Geometry: final body of the model. Coordinates: model frame, mm. A direction names the side the tool comes from. Coordinates: 2 decimals unless noted, no trailing zeros. Loops run counter-clockwise (first coordinate to the right, second up) from the corner with the lowest first, then second, coordinate; pieces in that order, holes last. Notation, with made-up numbers: (68, 7) -> (84, 7) arc R21 cw to (84, 12) -> close; hole circle Ø10 at (29, -8.5). An arc over 180 degrees is marked (long way). One line per item, written item: value. Start each with the question number.
Item 1: Section query C-C on y = 1.75. Return loops of the section in (x, z), then the cut area to 3 significant figures.
Item 2: Ray query, probe 1 along Z at (x, y) = (0.5, 3.5); probe 2 along Z at (x, y) = (1, 1.5); probe 3 along Y at (x, z) = (-1, -41.5). Return the intervals inside material, ascending. Write a range as from..to.
Item 3: Section query B-B on z = 0.5. Return loops of the section in (x, y) (3 decimals).
Item 4: Section query A-A on x = 0. Return loops of the section in (y, z) (3 decimals), then the cut area to 3 significant figures.
Item 5: Mould query, pull axis X, two halves, no side actions, for faces 4 (the flat face through (0, 2.468, 3)), 5 (the flat face through (0, 0, -45)), 6 (the cylindrical face through (2.6, -4.99, 1.97)). Classes: +X half, -X half, draft (parallel to the pull), parting line (faces both ways), or undercut.
Item 6: Contact query for flat-ended pins moving along their axis: pin 1 Ø6 at (x, z) = (-4, -38) entering from -Y; pin 2 Ø5 at (x, z) = (-0.5, -3.5) entering from +Y; pin 3 Ø5 at (y, z) = (-2.5, -38.5) entering from +X. Output: stop coordinate, or through.
Item 7: Set-up query: faces 1 (the flat face through (0, -2.468, 3)), 2 (the flat face through (0, 3, 4)), 3 (the flat face through (2.4, -2.4, 0)). Return all of +Z, -Z, +X, -X, +Y, -Y with unobstructed straight access to the full face (end or side cutting, diameter ignored); none if empty.
Item 8: Section query D-D on z = -9. Return loops of the section in (x, y), then the cut area to 3 significant figures.
from build123d import *

# Parameters (mm, degrees)
ESBO_O1_R                = 5.625
RESSALTO_EXTRUS_O1_DEPTH = 4
CORTE_EXTRUS_O1_DEPTH    = 2.5
ESBO_O3_R                = 3
RESSALTO_EXTRUS_O2_DEPTH = 45


with BuildPart() as part:
    # Esboço1 → Ressalto-extrusão1 (new body)
    with BuildSketch(Plane.XY):
        Circle(ESBO_O1_R)
    extrude(amount=RESSALTO_EXTRUS_O1_DEPTH)

    # Esboço2 → Corte-extrusão1 (cut)
    with BuildSketch(Plane.XY.offset(4)):
        Polygon((2.85, 0), (1.425, 2.468172401), (-1.425, 2.468172401), (-2.85, 0), (-1.425, -2.468172401), (1.425, -2.468172401), align=None)
    extrude(amount=-CORTE_EXTRUS_O1_DEPTH, mode=Mode.SUBTRACT)

    # Esboço3 → Ressalto-extrusão2 (add)
    with BuildSketch(Plane(origin=(0, 0, 0), x_dir=(-1, 0, 0), z_dir=(0, 0, -1))):
        with Locations(Location((0, 0, 0), (0, 0, 180))):
            Circle(ESBO_O3_R)
    extrude(amount=RESSALTO_EXTRUS_O2_DEPTH)


solid = part.part
Reply:
1. outline: (-5.35, 0) -> (-2.44, 0) -> (-2.44, -45) -> (2.44, -45) -> (2.44, 0) -> (5.35, 0) -> (5.35, 4) -> (1.84, 4) -> (1.84, 1.5) -> (-1.84, 1.5) -> (-1.84, 4) -> (-5.35, 4) -> close
1. area: 253 mm²
2. probe 1: z = 0..4
2. probe 2: z = -45..1.5
2. probe 3: y = -2.83..2.83
3. outline: circle Ø11.25 at (0, 0)
4. outline: (-5.625, 0) -> (-3, 0) -> (-3, -45) -> (3, -45) -> (3, 0) -> (5.625, 0) -> (5.625, 4) -> (2.468, 4) -> (2.468, 1.5) -> (-2.468, 1.5) -> (-2.468, 4) -> (-5.625, 4) -> close
4. area: 303 mm²
5. face 4: undercut
5. face 5: draft
5. face 6: parting line
6. pin 1: stops at y = -2.83
6. pin 2: stops at y = 3
6. pin 3: stops at x = 3
7. face 1: +Z
7. face 2: +Z, +X, -X, +Y, -Y
7. face 3: -Z
8. outline: circle Ø6 at (0, 0)
8. area: 28.3 mm²
